Geometry check sheet. Reference: the model listing, model coordinates, mm. A direction names the side the tool comes from. Coordinates: 2 decimals unless noted, no trailing zeros. Write each loop counter-clockwise with the first axis right and the second up, starting at its lowest first coordinate (ties: lowest second). Pieces come first, ordered by that corner, then holes. Notation, with made-up numbers: (-5, 34.25) -> (51, 34.25) arc R24 cw to (51, 60.25) -> close; hole circle Ø10 at (49, 73). An arc over 180 degrees is marked (long way). One line per question, with ' | ' between items.
```python
from build123d import *

# Parameters (mm, degrees)
BOSS_EXTRUDE1_DEPTH                       = 114.3
CHAMFER1_SIZE                             = 12.7
CSK_FOR_8_FLAT_HEAD_MACHINE_SCREW_2_COUNT = 2
CSK_FOR_8_FLAT_HEAD_MACHINE_SCREW_2_PITCH = 76.2
CSK_FOR_8_FLAT_HEAD_MACHINE_SCREW_3_COUNT = 2
CSK_FOR_8_FLAT_HEAD_MACHINE_SCREW_3_PITCH = 38.1
CSK_FOR_8_FLAT_HEAD_MACHINE_SCREW_4_COUNT = 2
CSK_FOR_8_FLAT_HEAD_MACHINE_SCREW_4_PITCH = 44.45


with BuildPart() as part:
    # Sketch2 → Boss-Extrude1 (new body)
    with BuildSketch(Plane.XY):
        Polygon((0, 0), (0, 50.8), (-3.175, 50.8), (-3.175, 3.175), (-50.8, 3.175), (-50.8, 0), align=None)
    extrude(amount=-BOSS_EXTRUDE1_DEPTH)

    # Chamfer1
    chamfer1_edges = [part.edges().sort_by_distance(p)[0] for p in [
        (-1.5875, 50.8, -114.3),
        (-50.8, 1.5875, -114.3),
        (-50.8, 1.5875, 0),
        (-1.5875, 50.8, 0),
    ]]
    chamfer(chamfer1_edges, length=CHAMFER1_SIZE)

    # Sketch4 → CSK for #8 Flat Head Machine Screw (100)1 (revolve, cut)
    with BuildSketch(Plane(origin=(-26.9875, 3.175, -95.25), x_dir=(0, 0, 1), z_dir=(1, 0, 0))):
        Polygon((0, 0), (0, 3.175), (2.45745, 3.175), (2.45745, 1.475934296), (4.2164, 0), align=None)
    csk_for_8_flat_head_machine_screw_100 = revolve(axis=Axis((-26.9875, 9.525, -95.25), (0, -1, 0)), mode=Mode.SUBTRACT)

    # CSK for _8 Flat Head Machine Screw _ 2: CSK for #8 Flat Head Machine Screw (100)1 ×2
    with Locations(*[(0, 0, i * CSK_FOR_8_FLAT_HEAD_MACHINE_SCREW_2_PITCH) for i in range(1, CSK_FOR_8_FLAT_HEAD_MACHINE_SCREW_2_COUNT)]):
        add(csk_for_8_flat_head_machine_screw_100, mode=Mode.SUBTRACT)

    # CSK for _8 Flat Head Machine Screw _ 3: CSK for #8 Flat Head Machine Screw (100)1 ×2
    with Locations(*[(0, 0, i * CSK_FOR_8_FLAT_HEAD_MACHINE_SCREW_3_PITCH) for i in range(1, CSK_FOR_8_FLAT_HEAD_MACHINE_SCREW_3_COUNT)]):
        add(csk_for_8_flat_head_machine_screw_100, mode=Mode.SUBTRACT)

    # CSK for _8 Flat Head Machine Screw _ 4: CSK for #8 Flat Head Machine Screw (100)1 ×2
    with Locations(*[(0, 0, -i * CSK_FOR_8_FLAT_HEAD_MACHINE_SCREW_4_PITCH) for i in range(1, CSK_FOR_8_FLAT_HEAD_MACHINE_SCREW_4_COUNT)]):
        add(csk_for_8_flat_head_machine_screw_100, mode=Mode.SUBTRACT)


solid = part.part
```
(1) Depth check by flat-ended pin: P1, Ø1.5, axis at x = -35, z = -80, coming from the +Y side (3 decimals); P2, Ø6, axis at y = 8.5, z = -47, coming from the -X side (3 decimals); P3, Ø5.5, axis at x = -26.99, z = -19.05, coming from the +Y side; P4, Ø5, axis at x = -37.5, z = -37, coming from the -Y side. Enter the tip coordinate at first touch or a pass-through.
Answers below:
P1: stops at y = 3.175 | P2: stops at x = -3.175 | P3: stops at y = 1.95 | P4: stops at y = 0
(2) Material ranges on line 1 (X direction, y = 1, z = -19); line 2 (Y direction, x = -47, z = -74) (3 decimals); line 3 (X direction, y = 11, z = -71) (3 decimals), recorded low to high.
Answers below:
line 1: x = -50.8 to -29.44, -24.53 to 0 | line 2: y = 0 to 3.175 | line 3: x = -3.175 to 0
(3) Cross-section at B-B (z = -30). Record the cut outline in (x, y) (3 decimals), plus the area to 4 significant figures.
Answers below:
outline: (-50.8, 0) -> (0, 0) -> (0, 50.8) -> (-3.175, 50.8) -> (-3.175, 3.175) -> (-50.8, 3.175) -> close | area: 312.5 mm²
(4) Cross-section at C-C (x = -14). Record the cut outline in (y, z) (3 decimals).
Answers below:
outline: (0, -114.3) -> (3.175, -114.3) -> (3.175, 0) -> (0, 0) -> close
(5) Cross-section at D-D (y = 28). Record the cut outline in (x, z) (3 decimals), plus the area to 3 significant figures.
Answers below:
outline: (-3.175, -114.3) -> (0, -114.3) -> (0, 0) -> (-3.175, 0) -> close | area: 363 mm²
(6) Draft check along X on faces 3 (the face through (-27.096, 0.861, -97.705)), 4 (the face through (-44.4, 1.6, -6.3)), 5 (the face through (-1.6, 44.4, -6.3)). Enter one of: pulls with the +X half, pulls with the -X half, needs draft (parallel to the pull), parting line crosses it, or undercut.
Answers below:
face 3: undercut | face 4: pulls with the -X half | face 5: needs draft
(7) Cross-section at A-A (z = -57.15). Record the cut outline in (x, y) (3 decimals), plus the area to 3 significant figures.
Answers below:
outline: (-50.8, 0) -> (-29.445, 0) -> (-29.445, 1.699) -> (-31.204, 3.175) -> (-50.8, 3.175) -> close; (-24.53, 0) -> (0, 0) -> (0, 50.8) -> (-3.175, 50.8) -> (-3.175, 3.175) -> (-22.771, 3.175) -> (-24.53, 1.699) -> close | area: 294 mm²
(8) Tool access check on faces 1 (the face through (-21, 3.175, -56)), 2 (the face through (-11, 2, -114.3)). Record the directions out of +Z, -Z, +X, -X, +Y, -Y that give a thin tool (end or side, any length) a straight path to the whole face; none if there is none.
Answers below:
face 1: +Z, -Z, -X, +Y | face 2: -Z, +X, -X, +Y, -Y
